Geometry check sheet. Reference: drawing and pictorial views, mm from the part's lowest x, y, z. A direction names the side the tool comes from. Round coordinates to 2 decimals unless told otherwise and drop trailing zeros. Write each loop counter-clockwise with the first axis right and the second up, starting at its lowest first coordinate (ties: lowest second). Pieces come first, ordered by that corner, then holes. Notation, with made-up numbers: (6.25, 16.25) - (62.25, 16.25) arc R16 cw to (62.25, 39.25) - close; hole circle Ø2 at (71, 56). An arc over 180 degrees is marked (long way). Return JSON: item names as keys, results as strings.
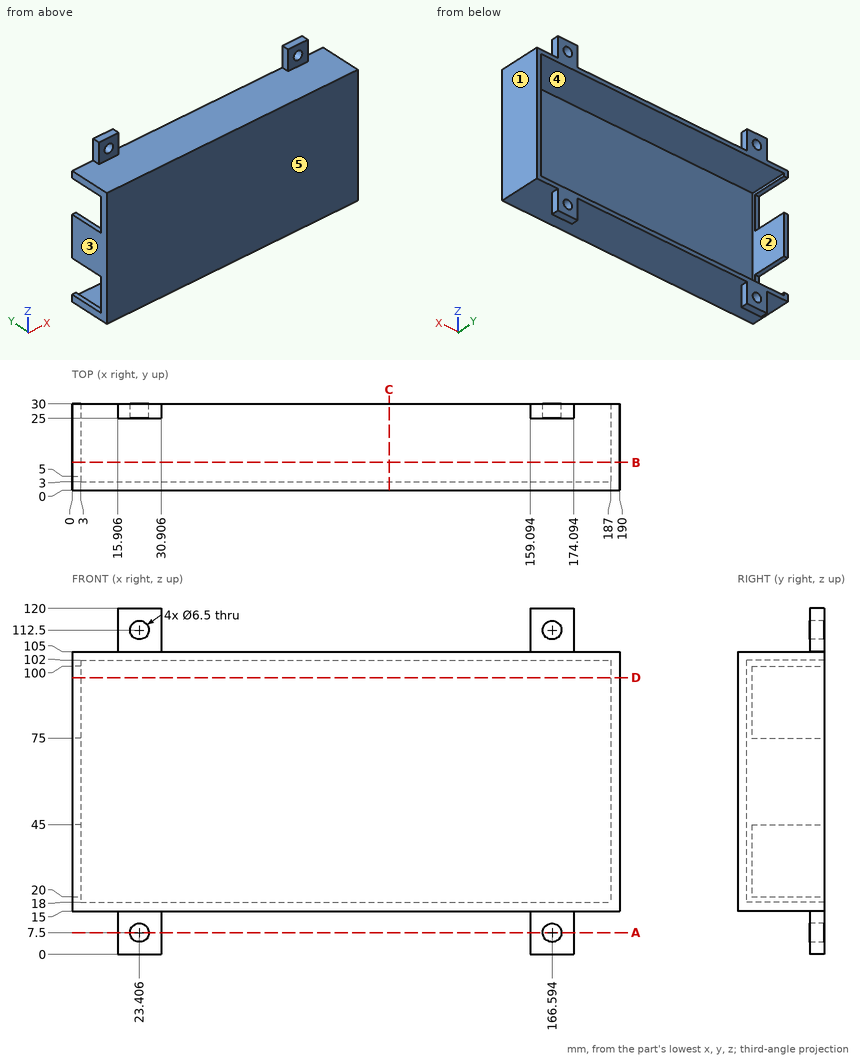
(1) Access from +Z, -Z, +X, -X, +Y, -Y to the whole of each face (thin tool, end or side, straight path). Record for the marked faces 4 and 5.
Response values:
{"face 4": "+Y", "face 5": "+Z, -Z, +X, -X, -Y"}
(2) Section check A-A, the plane z = 7.5. Enter the section's corners in (x, y).
Response values:
{"outline": "(15.91, 25) - (20.16, 25) - (20.16, 30) - (15.91, 30) - close; (26.66, 25) - (30.91, 25) - (30.91, 30) - (26.66, 30) - close; (159.09, 25) - (163.34, 25) - (163.34, 30) - (159.09, 30) - close; (169.84, 25) - (174.09, 25) - (174.09, 30) - (169.84, 30) - close"}
(3) Section check B-B, the plane y = 9.75. Enter the section's corners in (x, z).
Response values:
{"outline": "(0, 15) - (190, 15) - (190, 105) - (0, 105) - (0, 100) - (3, 100) - (3, 102) - (187, 102) - (187, 18) - (3, 18) - (3, 20) - (0, 20) - close; (0, 45) - (3, 45) - (3, 75) - (0, 75) - close"}
(4) Gauge pin test, flat ends, axial feed: pin 1 (8.5 mm diameter, centred on x = 166.59, z = 7.5, fed in from -Y); pin 2 (3.5 mm diameter, centred on x = 2, y = 11.5, fed in from +Z); pin 3 (4 mm diameter, centred on y = 27.5, z = 115, fed in from +X); pin 4 (5 mm diameter, centred on x = 23.41, z = 112.5, fed in from -Y). Record the tip position at first contact, or that the pin passes through.
Response values:
{"pin 1": "stops at y = 25", "pin 2": "stops at z = 105", "pin 3": "stops at x = 174.09", "pin 4": "passes through"}
(5) Section check D-D, the plane z = 96. Enter the section's corners in (x, y), plus the area to 3 significant figures.
Response values:
{"outline": "(0, 0) - (190, 0) - (190, 30) - (187, 30) - (187, 3) - (3, 3) - (3, 5) - (0, 5) - close", "area": "657 mm^2"}
(6) Material ranges on line 1 along X through (y, z) = (26.1, 7.5); line 2 along X through (y, z) = (19, 65); line 3 along Z through (x, y) = (138, 25.25), recorded low to high. Write a range as [from, to].
Response values:
{"line 1": "x = [15.91, 20.16], [26.66, 30.91], [159.09, 163.34], [169.84, 174.09]", "line 2": "x = [0, 3], [187, 190]", "line 3": "z = [15, 18], [102, 105]"}
(7) Release check for a two-part mould opening along X. For the marked faces 1, 2 and 3 record: pulls with the +X half, pulls with the -X half, needs draft (parallel to the pull), parting line crosses it, or undercut.
Response values:
{"face 1": "pulls with the +X half", "face 2": "undercut", "face 3": "pulls with the -X half"}
(8) Section check C-C, the plane x = 110. Enter the section's corners in (y, z), plus the area to 3 significant figures.
Response values:
{"outline": "(0, 15) - (30, 15) - (30, 18) - (3, 18) - (3, 102) - (30, 102) - (30, 105) - (0, 105) - close", "area": "432 mm^2"}
